from build123d import *

# Parameters (mm, degrees)
SKETCH1_R               = 1.6
BOSS_EXTRUDE1_DEPTH     = 70
SKETCH2_W               = 10
SKETCH2_H               = 0.35
CUT_EXTRUDE1_DEPTH      = 2.6
CUT_EXTRUDE1_DEPTH_BACK = 2.6
CHAMFER1_SIZE           = 0.1


with BuildPart() as part:
    # Sketch1 → Boss-Extrude1 (new body)
    with BuildSketch(Plane.XY):
        Circle(SKETCH1_R)
    extrude(amount=BOSS_EXTRUDE1_DEPTH)

    # Sketch2 → Cut-Extrude1 (cut, two sides)
    with BuildSketch(Plane(origin=(0, 0, 0), x_dir=(0, 0, -1), z_dir=(1, 0, 0))) as cut_extrude1_sk:
        with Locations((-5, 1.425)):
            Rectangle(SKETCH2_W, SKETCH2_H)
    extrude(amount=CUT_EXTRUDE1_DEPTH, mode=Mode.SUBTRACT)
    extrude(cut_extrude1_sk.sketch, amount=-CUT_EXTRUDE1_DEPTH_BACK, mode=Mode.SUBTRACT)

    # Chamfer1
    chamfer1_edges = [part.edges().sort_by_distance(p)[0] for p in [
        (-1.6, 0, 70),
        (-0.693542087, -1.441873564, 0),
    ]]
    chamfer(chamfer1_edges, length=CHAMFER1_SIZE)


solid = part.part
Read the model definition and answer for the solid it produces. Units are mm, in the model's axes. A direction names the side the tool comes from. Coordinates: 2 decimals unless noted, no trailing zeros. Order: outer loops, then holes, each group sorted by start corner. A loop starts at its lowest first (then second) coordinate and runs counter-clockwise, first axis right, second up. Notation, with made-up numbers: M 1.25,-32 L 35.25,-32 A12 ccw 35.25,-11 Z; hole C 26,-12.5 d1. An arc over 180 degrees is marked long. Put each result on its own line as item: value. Start each with the question number.
Item 1: Section C-C, the plane z = 31 is taken. Determine the outline of the cut face in (x, y), plus the area to 3 significant figures.
Item 2: Consider probe 1 along Y at (x, z) = (-1.25, 49); probe 2 along Z at (x, y) = (0, 1.35); probe 3 along Y at (x, z) = (0.15, 23). Determine where each line is inside the solid, lowest interval first. Write a range as [from, to].
Item 3: Section B-B, the plane z = 4.5 is taken. Determine the outline of the cut face in (x, y), plus the area to 3 significant figures.
Item 4: Given pin 1 Ø1 at (x, z) = (0, 3) entering from +Y; pin 2 Ø1 at (x, z) = (-1, 40) entering from -Y, each flat-ended and moving along its own axis, determine where each tip first touches the part or whether it passes through.
Item 5: For faces 1 (the face through (0, 0, 70)), 2 (the face through (0, 1.25, 5)), determine the directions among +Z, -Z, +X, -X, +Y, -Y from which every point of the face is accessible in a straight line to the end or side of a thin tool.
Item 6: Section A-A, the plane x = 0 is taken. Determine the outline of the cut face in (y, z).
Computed:
1. outline: C 0,0 d3.2
1. area: 8.04 mm2
2. probe 1: y = [-1, 1]
2. probe 2: z = [10, 70]
2. probe 3: y = [-1.59, 1.59]
3. outline: M -1,1.25 A1.6 ccw long 1,1.25 Z
3. area: 7.57 mm2
4. pin 1: stops at y = 1.25
4. pin 2: stops at y = -1.52
5. face 1: +Z, +X, -X, +Y, -Y
5. face 2: -Z, +X, -X, +Y
6. outline: M -1.6,0.1 L -1.5,0 L 1.25,0 L 1.25,10 L 1.6,10 L 1.6,69.9 L 1.5,70 L -1.5,70 L -1.6,69.9 Z
